from build123d import *

# Parameters (mm, degrees)
SKETCH_1_W          = 15
SKETCH_1_H          = 15
EXTRUDE_1_DEPTH     = 15
SKETCH_2_W          = 8
SKETCH_2_H          = 8
CUT_EXTRUDE_1_DEPTH = 17.5
SKETCH_3_R          = 1.65
CUT_EXTRUDE_2_DEPTH = 17.5
SKETCH_5_W          = 15
SKETCH_5_H          = 15
EXTRUDE_2_DEPTH     = 35
SKETCH_6_W          = 28
SKETCH_6_H          = 25
EXTRUDE_3_DEPTH     = 2


with BuildPart() as part:
    # 草图1 → 凸台-拉伸1 (new body)
    with BuildSketch(Plane(origin=(0, 0, 0), x_dir=(1, 0, 0), z_dir=(0, 1, 0))):
        Rectangle(SKETCH_1_W, SKETCH_1_H)
    extrude(amount=-EXTRUDE_1_DEPTH)

    # 草图2 → 切除-拉伸1 (cut, symmetric)
    with BuildSketch(Plane.XY):
        with Locations((0, -11)):
            Rectangle(SKETCH_2_W, SKETCH_2_H)
    extrude(amount=CUT_EXTRUDE_1_DEPTH, both=True, mode=Mode.SUBTRACT)

    # 草图3 → 切除-拉伸2 (cut, symmetric)
    with BuildSketch(Plane(origin=(0, 0, 0), x_dir=(1, 0, 0), z_dir=(0, 1, 0))):
        with Locations(Location((0, 0, 0), (0, 0, 270))):
            Circle(SKETCH_3_R)
    extrude(amount=CUT_EXTRUDE_2_DEPTH, both=True, mode=Mode.SUBTRACT)

    # 草图5 → 凸台-拉伸2 (add)
    with BuildSketch(Plane(origin=(7.5, 0, 0), x_dir=(0, 0, -1), z_dir=(1, 0, 0))):
        with Locations((0, -7.5)):
            Rectangle(SKETCH_5_W, SKETCH_5_H)
    extrude(amount=EXTRUDE_2_DEPTH)

    # 草图6 → 凸台-拉伸3 (add)
    with BuildSketch(Plane(origin=(42.5, 0, 0), x_dir=(0, 0, -1), z_dir=(1, 0, 0))):
        with Locations((0, -2.5)):
            Rectangle(SKETCH_6_W, SKETCH_6_H)
    extrude(amount=-EXTRUDE_3_DEPTH)


solid = part.part
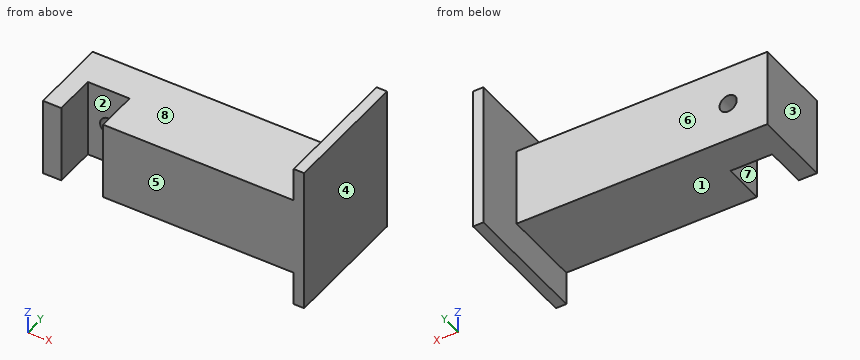
CAD build for the part. Positions are in the model's coordinates, mm. Face numbers are marked on the shaded views. A direction names the side the tool comes from. Give positions to 0.01 mm unless a question says otherwise; leave off trailing zeros. Write each loop counter-clockwise with the first axis right and the second up, starting at its lowest first coordinate (ties: lowest second). Pieces come first, ordered by that corner, then holes. Notation, with made-up numbers: (81, 83.25) - (87, 83.25) arc R11 ccw to (87, 88.25) - close; hole circle Ø4 at (68.25, 51.25). An arc over 180 degrees is marked (long way). Put each result on its own line as item: value.
(1) Drop flat-ended pins along their axis: pin 1 Ø6 at (x, y) = (34.5, -8.5) entering from -Z; pin 2 Ø4.5 at (x, z) = (0, 0) entering from -Y; pin 3 Ø1.5 at (x, z) = (8.5, -4.5) entering from +Y; pin 4 Ø1 at (x, z) = (1.5, 9.5) entering from +Y. Give the stop position or say it passes through.
Working result:
pin 1: z = -7.5
pin 2: y = -7
pin 3: y = 0
pin 4: through
(2) Pull direction X, two halves, no side cores. Call the marked faces 1, 2, 3 and 4: released by +X, released by -X, zero draft, split by the parting line, or undercut.
Working result:
face 1: zero draft
face 2: undercut
face 3: released by -X
face 4: released by +X
(3) Saw through at D-D (y = -11). List the corners of the cut face in (x, z).
Working result:
outline: (-7.5, -7.5) - (-4, -7.5) - (-4, 7.5) - (-7.5, 7.5) - close; (4, -7.5) - (40.5, -7.5) - (40.5, -14) - (42.5, -14) - (42.5, 14) - (40.5, 14) - (40.5, 7.5) - (4, 7.5) - close
(4) Saw through at B-B (z = 0). List the corners of the cut face in (x, y).
Working result:
outline: (-7.5, -15) - (-4, -15) - (-4, -7) - (-1.65, -7) - (-1.65, 0) - (-7.5, 0) - close; (1.65, -7) - (4, -7) - (4, -15) - (42.5, -15) - (42.5, 10) - (40.5, 10) - (40.5, 0) - (1.65, 0) - close
(5) Saw through at A-A (y = -6). List the corners of the cut face in (x, z).
Working result:
outline: (-7.5, -7.5) - (40.5, -7.5) - (40.5, -14) - (42.5, -14) - (42.5, 14) - (40.5, 14) - (40.5, 7.5) - (-7.5, 7.5) - close; hole circle Ø3.3 at (0, 0)
(6) Tool access for the marked faces 5, 6, 7 and 8: list every direction of +Z, -Z, +X, -X, +Y, -Y with a clear straight run to the whole face (end or side of a thin tool).
Working result:
face 5: +Z, -Z, +X, -X, -Y
face 6: +Z, -Z, -X, +Y
face 7: +Z, -Z, -Y
face 8: +Z, -X, +Y, -Y
(7) Wall check: L1, parallel to X at y = -4.5, z = 0; L2, parallel to X at y = -10, z = 5; L3, parallel to X at y = 6.75, z = 10.5. Give the ranges that are in metal, low to high.
Working result:
L1: -7.5 to -1.65, 1.65 to 42.5
L2: -7.5 to -4, 4 to 42.5
L3: 40.5 to 42.5
(8) Saw through at C-C (x = 0). List the corners of the cut face in (y, z), then the cut area to 3 significant figures.
Working result:
outline: (-7, -7.5) - (0, -7.5) - (0, -1.65) - (-7, -1.65) - close; (-7, 1.65) - (0, 1.65) - (0, 7.5) - (-7, 7.5) - close
area: 81.9 mm^2
